Geometry check sheet. Reference: the model listing, model coordinates, mm. Face numbers are marked on the shaded views. A direction names the side the tool comes from. Give positions to 0.01 mm unless a question says otherwise; leave off trailing zeros. Order: outer loops, then holes, each group sorted by start corner. A loop starts at its lowest first (then second) coordinate and runs counter-clockwise, first axis right, second up. Notation, with made-up numbers: M -7.5,-23.5 L 29.5,-23.5 A6 cw 29.5,-12.5 Z; hole C 32,8 d3. An arc over 180 degrees is marked long. One line per question, with ' | ' between items. Start each with the question number.
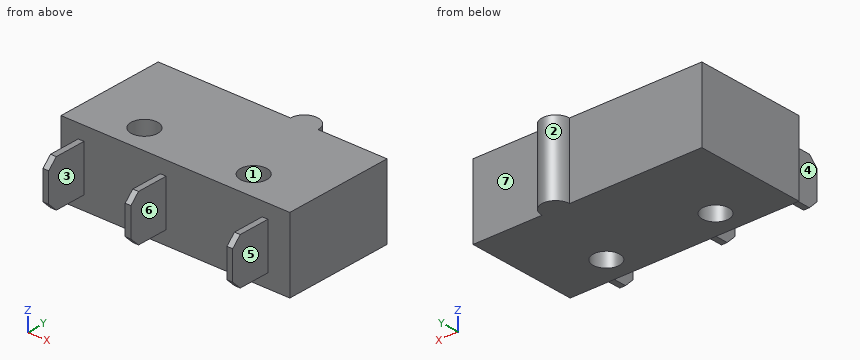
from build123d import *

# Parameters (mm, degrees)
SKETCH_R     = 1.15
PAD_DEPTH    = 6.4
SKETCH001_W  = 0.5
SKETCH001_H  = 4
PAD001_DEPTH = 3.5
CHAMFER_SIZE = 0.75


with BuildPart() as part:
    # Sketch → Pad (new body)
    with BuildSketch(Plane.XY):
        with BuildLine():
            Line((0, 0), (19.9, 0))
            Line((19.9, 0), (19.9, 9.65))
            Line((19.9, 9.65), (13.9, 9.65))
            ThreePointArc((13.9, 9.65), (12.7, 10.85), (11.5, 9.65))
            Line((11.5, 9.65), (0, 9.65))
            Line((0, 9.65), (0, 0))
        make_face()
        with Locations((5.2, 2.35)):
            Circle(SKETCH_R, mode=Mode.SUBTRACT)
        with Locations((14.7, 2.35)):
            Circle(SKETCH_R, mode=Mode.SUBTRACT)
    extrude(amount=PAD_DEPTH)

    # Sketch001 → Pad001 (join)
    with BuildSketch(Plane.XZ):
        with Locations((1.75, 3.2)):
            Rectangle(SKETCH001_W, SKETCH001_H)
        with Locations((8.9, 3.2)):
            Rectangle(SKETCH001_W, SKETCH001_H)
        with Locations((17.75, 3.2)):
            Rectangle(SKETCH001_W, SKETCH001_H)
    extrude(amount=PAD001_DEPTH)

    # Chamfer
    chamfer_edges = [part.edges().sort_by_distance(p)[0] for p in [
        (17.75, -3.5, 5.2),
        (17.75, -3.5, 1.2),
        (1.75, -3.5, 1.2),
        (1.75, -3.5, 5.2),
        (8.9, -3.5, 5.2),
        (8.9, -3.5, 1.2),
    ]]
    chamfer(chamfer_edges, length=CHAMFER_SIZE)


solid = part.part
Item 1: Cross-section at A-A, the plane x = 5.2. Record the cut outline in (y, z), plus the area to 3 significant figures.
Item 2: Set-up check for the marked faces 5, 6 and 7: record each of +Z, -Z, +X, -X, +Y, -Y from which the full face is reachable in a straight line by a thin tool's end or side.
Item 3: Cross-section at C-C, the plane y = 2.35. Record the cut outline in (x, z), plus the area to 3 significant figures.
Item 4: Cross-section at B-B, the plane z = 5.5. Record the cut outline in (x, y), plus the area to 3 significant figures.
Item 5: Depth check by flat-ended pin: pin 1 (1.8 mm diameter, centred on x = 16.5, z = 4, fed in from +Y); pin 2 (1.9 mm diameter, centred on x = 13, z = 4.5, fed in from -Y); pin 3 (1 mm diameter, centred on y = -2.5, z = 4, fed in from -X). Enter the tip coordinate at first touch or a pass-through.
Item 6: Cross-section at D-D, the plane z = 1.5. Record the cut outline in (x, y), plus the area to 3 significant figures.
Item 7: Mould release check, pull along X, two halves, no side actions. Record for the marked faces 1, 2, 3 and 4: released by +X, released by -X, zero draft, split by the parting line, or undercut.
Item 8: Material ranges on line 1 along X through (y, z) = (-2.5, 2.5); line 2 along Y through (x, z) = (14.7, 4.5); line 3 along X through (y, z) = (9.75, 4.5), recorded low to high.
Outcome:
1) outline: M 0,0 L 1.2,0 L 1.2,6.4 L 0,6.4 Z; M 3.5,0 L 9.65,0 L 9.65,6.4 L 3.5,6.4 Z | area: 47.0 mm²
2) face 5: +Z, -Z, +X, -Y | face 6: +Z, -Z, -Y | face 7: +Z, -Z, +X, +Y
3) outline: M 0,0 L 4.05,0 L 4.05,6.4 L 0,6.4 Z; M 6.35,0 L 13.55,0 L 13.55,6.4 L 6.35,6.4 Z; M 15.85,0 L 19.9,0 L 19.9,6.4 L 15.85,6.4 Z | area: 97.9 mm²
4) outline: M 0,0 L 19.9,0 L 19.9,9.65 L 13.9,9.65 A1.2 ccw 11.5,9.65 L 0,9.65 Z; hole C 5.2,2.35 d2.3; hole C 14.7,2.35 d2.3 | area: 186 mm²
5) pin 1: stops at y = 9.65 | pin 2: stops at y = 0 | pin 3: stops at x = 1.5
6) outline: M 0,0 L 1.5,0 L 1.5,-3.05 L 2,-3.05 L 2,0 L 8.65,0 L 8.65,-3.05 L 9.15,-3.05 L 9.15,0 L 17.5,0 L 17.5,-3.05 L 18,-3.05 L 18,0 L 19.9,0 L 19.9,9.65 L 13.9,9.65 A1.2 ccw 11.5,9.65 L 0,9.65 Z; hole C 5.2,2.35 d2.3; hole C 14.7,2.35 d2.3 | area: 191 mm²
7) face 1: undercut | face 2: split by the parting line | face 3: undercut | face 4: released by -X
8) line 1: x = 1.5 to 2, 8.65 to 9.15, 17.5 to 18 | line 2: y = 0 to 1.2, 3.5 to 9.65 | line 3: x = 11.5 to 13.9
